Input: part model. Units: mm. Frame: model coordinates. A direction names the side the tool comes from. Coordinates: 2 decimals unless noted, no trailing zeros. Order: outer loops, then holes, each group sorted by start corner. A loop starts at its lowest first (then second) coordinate and runs counter-clockwise, first axis right, second up.
Autodesk Inventor part; units mm, degrees
ref_plane "YZ Plane" through (0, 0, 0) normal (1, 0, 0) x (0, 1, 0)
ref_plane "XZ Plane" through (0, 0, 0) normal (0, 1, 0) x (-1, 0, 0)
ref_plane "XY Plane" through (0, 0, 0) normal (0, 0, 1) x (1, 0, 0)
sketch "Sketch1" plane through (0, 0, 0) normal (0, 0, 1) x (1, 0, 0)
  line L0 (0, 0) -> (38.1, 0)
  line L1 (38.1, 0) -> (38.1, 25.4)
  line L2 (38.1, 25.4) -> (0, 25.4)
  line L3 (0, 25.4) -> (0, 0)
  circle A0 centre (6.35, 12.7) radius 2.0701
  circle A1 centre (31.75, 12.7) radius 2.0701
  dimension "d0" = 38.1
  dimension "d1" = 25.4
  dimension "d2" = 4.1402
  dimension "d3" = 12.7
  dimension "d4" = 6.35
  dimension "d7" = 25.4
extrude "Plate1" add sketch "Sketch1" along normal blind 3.175
sketch "Sketch2" plane through (0, 22.225, 0) normal (0, 1, 0) x (-1, 0, 0)
  line L0 (-38.1, 0) -> (0, 0)
  line L1 (0, 0) -> (0, 44.45)
  line L2 (0, 44.45) -> (-38.1, 44.45)
  line L3 (-38.1, 44.45) -> (-38.1, 0)
edge flange "Flange1" height 44.45 angle 90 thickness 3.175 bend radius 1.27 thickness toward (0, 1, 0) relief tear relief width 3.175 relief depth 1.5875 edges at (19.05, 25.4, 3.175) wall of the first edge with corners at (38.1, 22.225, 0) (0, 22.225, 0) (0, 22.225, 44.45) (38.1, 22.225, 44.45)
bend "Bend1"
corner "Corner1"
sketch "Sketch3" plane through (0, 25.4, 44.45) normal (0, 1, 0) x (1, 0, 0)
  line L0 (38.1, 40.005) -> (0, 40.005)
  line L1 (38.1, 40.005) -> (38.1, 0)
  line L2 (28.575, 33.655) -> (9.525, 33.655) construction
  line L3 (9.525, 33.655) -> (9.525, 0.381) construction
  line L4 (9.525, 0.381) -> (28.575, 0.381) construction
  line L5 (28.575, 0.381) -> (28.575, 33.655) construction
  line L6 (28.575, 5.969) -> (9.525, 5.969) construction
  circle A0 centre (25.4, 5.969) radius 2.413
  line L7 (19.05, 0.381) -> (19.05, 33.655) construction
  circle A1 centre (12.7, 5.969) radius 2.413
  line L8 (28.575, 17.018) -> (9.525, 17.018) construction
  circle A2 centre (25.4, 28.067) radius 2.413
  circle A3 centre (12.7, 28.067) radius 2.413
  point P0 (0, 44.45)
  dimension "d23" = 19.05
  dimension "d24" = 33.274
  dimension "d25" = 5.588
  dimension "d26" = 3.175
  dimension "d27" = 4.826
  dimension "d28" = 9.525
  dimension "d29" = 6.35
extrude "Cut1" cut sketch "Sketch3" against normal blind 3.175
equation "\"d28\" = -0.5 * d23 + 0.5 * d0"
equation "\"d30\" = Thickness"
equation "\"d13\" = BendReliefWidth"
equation "\"d14\" = BendReliefDepth"
equation "\"d15\" = MinimumRemnant"
equation "\"d16\" = BendRadius"
equation "\"d20\" = CornerReliefSize"
equation "\"d21\" = GapSize"
equation "\"d22\" = JacobiRadiusSize"
equation "\"BendRadius\" = Thickness"
equation "\"BendReliefWidth\" = Thickness"
equation "\"BendReliefDepth\" = 0.5 * Thickness"
equation "\"CornerReliefSize\" = 4 * Thickness"
equation "\"MinimumRemnant\" = 2 * Thickness"
equation "\"TransitionRadius\" = BendRadius"
equation "\"JacobiRadiusSize\" = BendRadius"
equation "\"GapSize\" = Thickness"
equation "\"d12\" = BendRadius"
properties part number "Pneumatic Piston Back Flange (Custom)" material "Aluminum 6061"
Item 1: Access query for faces 1 (the face through (19, 11, 3.175)), 2 (the face through (19, 24, 44.45)). Directions: +Z, -Z, +X, -X, +Y, -Y. A direction counts if a zero-diameter tool reaches every point of the face in a straight line with its end or side. Return the directions, or none.
Response values:
face 1: +Z, +X, -X, -Y
face 2: +Z, +X, -X, +Y, -Y
Item 2: Ray query, probe 1 along Z at (x, y) = (29, 16.75) (3 decimals); probe 2 along Y at (x, z) = (31.75, 1.45); probe 3 along Z at (x, y) = (25.4, 23.8). Return the intervals inside material, ascending.
Response values:
probe 1: z = 0 to 3.175
probe 2: y = 0 to 10.63, 14.77 to 24.24
probe 3: z = 1.03 to 13.97, 18.8 to 36.07, 40.89 to 44.45
Item 3: Cut plane D-D on x = 6.35. Return loops of the section in (y, z) (3 decimals).
Response values:
outline: (0, 0) - (10.63, 0) - (10.63, 3.175) - (0, 3.175) - close; (14.77, 0) - (20.955, 0) arc R4.445 ccw to (25.4, 4.445) - (25.4, 44.45) - (22.225, 44.45) - (22.225, 4.445) arc R1.27 cw to (20.955, 3.175) - (14.77, 3.175) - close
Item 4: Draft query along Z for faces 3 (the face through (29.68, 12.61, 1.57)), 4 (the face through (12.18, 23.83, 18.74)), 5 (the face through (12.39, 23.83, 36.09)), 6 (the face through (18.783, 21.863, 3.557)). Return one class per face: pulls with the +Z half, pulls with the -Z half, needs draft (parallel to the pull), parting line crosses it, or undercut.
Response values:
face 3: needs draft
face 4: undercut
face 5: undercut
face 6: pulls with the +Z half
Item 5: Cut plane A-A on y = 12.7. Return loops of the section in (x, z) (3 decimals).
Response values:
outline: (0, 0) - (4.28, 0) - (4.28, 3.175) - (0, 3.175) - close; (8.42, 0) - (29.68, 0) - (29.68, 3.175) - (8.42, 3.175) - close; (33.82, 0) - (38.1, 0) - (38.1, 3.175) - (33.82, 3.175) - close
Item 6: Cut plane B-B on x = 25.4. Return loops of the section in (y, z) (3 decimals), then the cut area to 3 significant figures.
Response values:
outline: (0, 0) - (20.955, 0) arc R4.445 ccw to (25.4, 4.445) - (25.4, 13.97) - (22.225, 13.97) - (22.225, 4.445) arc R1.27 cw to (20.955, 3.175) - (0, 3.175) - close; (22.225, 18.796) - (25.4, 18.796) - (25.4, 36.068) - (22.225, 36.068) - close; (22.225, 40.894) - (25.4, 40.894) - (25.4, 44.45) - (22.225, 44.45) - close
area: 177 mm2
Item 7: Cut plane C-C on z = 18. Return loops of the section in (x, y) (3 decimals).
Response values:
outline: (0, 22.225) - (10.909, 22.225) - (10.909, 25.4) - (0, 25.4) - close; (14.491, 22.225) - (23.609, 22.225) - (23.609, 25.4) - (14.491, 25.4) - close; (27.191, 22.225) - (38.1, 22.225) - (38.1, 25.4) - (27.191, 25.4) - close
Item 8: Pin query (flat end, axial travel): pin 1 Ø5 at (x, z) = (29, 16) entering from -Y (3 decimals); pin 2 Ø3 at (x, y) = (13, 14.5) entering from +Z (3 decimals); pin 3 Ø3 at (x, z) = (12.7, 16.383) entering from -Y. Return the tip coordinate at first contact, or that it passes through.
Response values:
pin 1: stops at y = 22.225
pin 2: stops at z = 3.175
pin 3: passes through
